Verification items for the finished model (mm, model axes). Face numbers are marked on the shaded views. A direction names the side the tool comes from. Give positions to 0.01 mm unless a question says otherwise; leave off trailing zeros. Order: outer loops, then holes, each group sorted by start corner. A loop starts at its lowest first (then second) coordinate and runs counter-clockwise, first axis right, second up.
from build123d import *

# Parameters (mm, degrees)
SKETCH1_R                            = 17.5
BOSS_EXTRUDE1_DEPTH                  = 20
SKETCH2_R                            = 12
CUT_EXTRUDE1_DEPTH                   = 18
SKETCH2_3_R                          = 15.5
SKETCH2_3_R_2                        = 12
CUT_EXTRUDE2_DEPTH                   = 5
BOSS_EXTRUDE2_REACH                  = 33.82
BOSS_EXTRUDE2_END_RADIUS             = 12
BOSS_EXTRUDE2_DIRECTION_2_REACH      = 33.82
BOSS_EXTRUDE2_DIRECTION_2_END_RADIUS = 12
SKETCH5_W                            = 7
SKETCH5_H                            = 8.6
CUT_EXTRUDE3_DEPTH                   = 18
F_4_0MM_DOWEL_HOLE1_D                = 4
F_4_0MM_DOWEL_HOLE1_ON_FACE_2_D      = 4


with BuildPart() as part:
    # Sketch1 → Boss-Extrude1 (new body)
    with BuildSketch(Plane(origin=(0, 0, 0), x_dir=(1, 0, 0), z_dir=(0, 1, 0))):
        with Locations(Location((0, 0, 0), (0, 0, 270))):
            Circle(SKETCH1_R)
    extrude(amount=BOSS_EXTRUDE1_DEPTH)

    # Sketch2 → Cut-Extrude1 (cut)
    with BuildSketch(Plane(origin=(0, 20, 0), x_dir=(1, 0, 0), z_dir=(0, 1, 0))):
        with Locations(Location((0, 0, 0), (0, 0, 270))):
            Circle(SKETCH2_R)
    extrude(amount=-CUT_EXTRUDE1_DEPTH, mode=Mode.SUBTRACT)

    # Sketch2<3> → Cut-Extrude2 (cut)
    with BuildSketch(Plane(origin=(0, 20, 0), x_dir=(1, 0, 0), z_dir=(0, 1, 0))):
        with Locations(Location((0, 0, 0), (0, 0, 270))):
            Circle(SKETCH2_3_R)
        with Locations(Location((0, 0, 0), (0, 0, 270))):
            Circle(SKETCH2_3_R_2, mode=Mode.SUBTRACT)
    extrude(amount=-CUT_EXTRUDE2_DEPTH, mode=Mode.SUBTRACT)

    # Boss-Extrude2: up to this cylinder (the profile starts inside it)
    boss_extrude2_end = Plane(origin=(0, 8.116384, 0), z_dir=(0, 1, 0)) * Cylinder(BOSS_EXTRUDE2_END_RADIUS, 92.64, mode=Mode.PRIVATE)
    # Sketch3 → Boss-Extrude2 (add, up to the surface)
    with BuildSketch(Plane.XY, mode=Mode.PRIVATE) as boss_extrude2_sk1:
        with BuildLine():
            Line((-2.5, 8.050510257), (-2.5, 2))
            Line((-2.5, 2), (2.5, 2))
            Line((2.5, 2), (2.5, 8.050510257))
            ThreePointArc((2.5, 8.050510257), (0, 14), (-2.5, 8.050510257))
        make_face()
    boss_extrude2_tool1 = extrude(boss_extrude2_sk1.sketch, amount=BOSS_EXTRUDE2_REACH, mode=Mode.PRIVATE) & boss_extrude2_end
    add(boss_extrude2_tool1.solids().sort_by_distance((0, 8.116384, 0))[0])

    # Boss-Extrude2 direction 2: up to this cylinder (the profile starts inside it)
    boss_extrude2_direction_2_end = Plane(origin=(0, 8.116384, 0), z_dir=(0, 1, 0)) * Cylinder(BOSS_EXTRUDE2_DIRECTION_2_END_RADIUS, 92.64, mode=Mode.PRIVATE)
    # Sketch3 → Boss-Extrude2 direction 2 (add, up to the surface)
    with BuildSketch(Plane.XY, mode=Mode.PRIVATE) as boss_extrude2_direction_2_sk1:
        with BuildLine():
            Line((-2.5, 8.050510257), (-2.5, 2))
            Line((-2.5, 2), (2.5, 2))
            Line((2.5, 2), (2.5, 8.050510257))
            ThreePointArc((2.5, 8.050510257), (0, 14), (-2.5, 8.050510257))
        make_face()
    boss_extrude2_direction_2_tool1 = extrude(boss_extrude2_direction_2_sk1.sketch, amount=-BOSS_EXTRUDE2_DIRECTION_2_REACH, mode=Mode.PRIVATE) & boss_extrude2_direction_2_end
    add(boss_extrude2_direction_2_tool1.solids().sort_by_distance((0, 8.116384, 0))[0])

    # Sketch5 → Cut-Extrude3 (cut)
    with BuildSketch(Plane(origin=(0, 20, 0), x_dir=(1, 0, 0), z_dir=(0, 1, 0))):
        Rectangle(SKETCH5_W, SKETCH5_H)
    extrude(amount=-CUT_EXTRUDE3_DEPTH, mode=Mode.SUBTRACT)

    # Ø4.0mm Dowel Hole1 (through all)
    with Locations(Plane(origin=(0, 0, 0), x_dir=(0, 0, -1), z_dir=(0, -1, 0))):
        with Locations((0, 0)):
            Hole(F_4_0MM_DOWEL_HOLE1_D / 2)

    # Ø4.0mm Dowel Hole1 on face 2 (through all)
    with Locations(Plane.ZX.offset(2)):
        with Locations((0, 0)):
            Hole(F_4_0MM_DOWEL_HOLE1_ON_FACE_2_D / 2)


solid = part.part
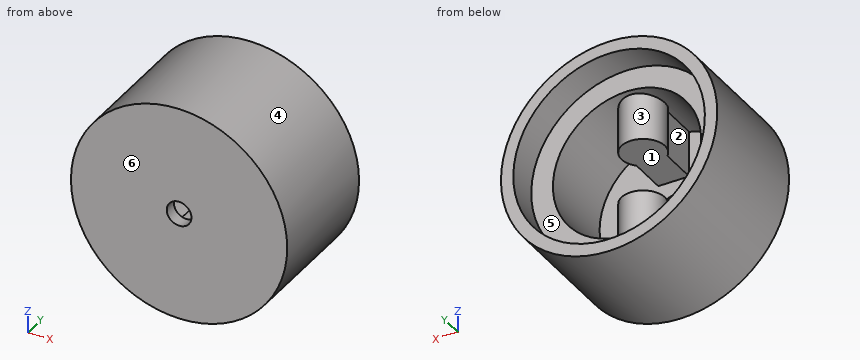
(1) Section check B-B, the plane z = 0. Enter the section's corners in (x, y), then the cut area to 3 significant figures.
Solved:
outline: (-17.5, 0) - (-2, 0) - (-2, 2) - (-12, 2) - (-12, 15) - (-15.5, 15) - (-15.5, 20) - (-17.5, 20) - close; (2, 0) - (17.5, 0) - (17.5, 20) - (15.5, 20) - (15.5, 15) - (12, 15) - (12, 2) - (2, 2) - close
area: 225 mm2
(2) Scan lines: line 1 (X direction, y = 0.8, z = 0); line 2 (X direction, y = 2.75, z = 5); line 3 (X direction, y = 13, z = -7). Record each from-to range of solid material in increasing order.
Solved:
line 1: x = -17.5 to -2, 2 to 17.5
line 2: x = -16.77 to -10.91, -2.5 to 2.5, 10.91 to 16.77
line 3: x = -16.04 to -9.75, -2.45 to 2.45, 9.75 to 16.04
(3) Go/stop test with flat-tipped pins: pin 1 (1 mm diameter, centred on x = -5, y = 6.5, fed in from +Z); pin 2 (11.5 mm diameter, centred on x = 5.5, z = -2.5, fed in from +Y); pin 3 (5 mm diameter, centred on y = 4, z = 10, fed in from -X); pin 4 (2.5 mm diameter, centred on x = 0, z = 0, fed in from +Y). Record where each tip stops, or that it passes through.
Solved:
pin 1: stops at z = 16.91
pin 2: stops at y = 14
pin 3: stops at x = -15.81
pin 4: passes through
(4) Section check A-A, the plane x = 0. Enter the section's corners in (y, z), then the cut area to 3 significant figures.
Solved:
outline: (0, -17.5) - (20, -17.5) - (20, -15.5) - (15, -15.5) - (15, -12) - (14, -12) - (14, -4.3) - (2, -4.3) - (2, -2) - (0, -2) - close; (0, 2) - (2, 2) - (2, 4.3) - (14, 4.3) - (14, 12) - (15, 12) - (15, 15.5) - (20, 15.5) - (20, 17.5) - (0, 17.5) - close
area: 410 mm2
(5) Set-up check for the marked faces 1 and 2: record each of +Z, -Z, +X, -X, +Y, -Y from which the full face is reachable in a straight line by a thin tool's end or side.
Solved:
face 1: +Y
face 2: none
(6) Release check for a two-part mould opening along X. For the marked faces 3, 4, 5 and 6 record: pulls with the +X half, pulls with the -X half, needs draft (parallel to the pull), parting line crosses it, or undercut.
Solved:
face 3: undercut
face 4: parting line crosses it
face 5: undercut
face 6: needs draft
(7) Section check C-C, the plane y = 4.25. Enter the section's corners in (x, z), then the cut area to 3 significant figures.
Solved:
outline: circle Ø35 at (0, 0); hole (-2.5, -11.74) - (-2.5, -4.3) - (2.5, -4.3) - (2.5, -11.74) arc R12 ccw to (2.5, 11.74) - (2.5, 4.3) - (-2.5, 4.3) - (-2.5, 11.74) arc R12 ccw to start
area: 586 mm2
(8) Section check D-D, the plane z = -14. Enter the section's corners in (x, y).
Solved:
outline: (-10.5, 0) - (10.5, 0) - (10.5, 20) - (6.65, 20) - (6.65, 15) - (-6.65, 15) - (-6.65, 20) - (-10.5, 20) - close
